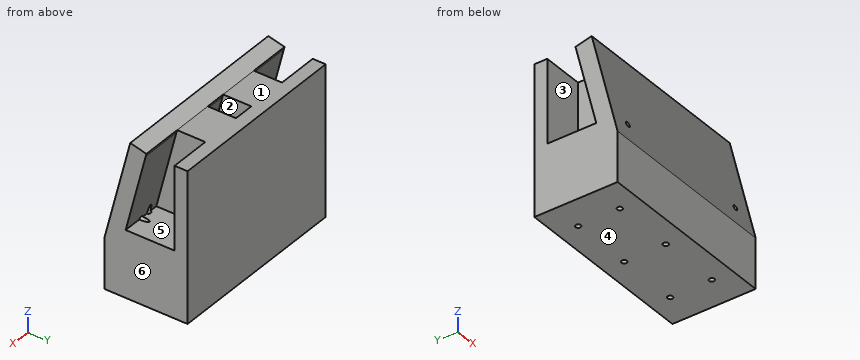
Autodesk Inventor part; units mm, degrees
ref_plane "作業平面1" through (45, 0, 0) normal (-1, 0, 0) x (0, 0, 1)
ref_plane "YZ Plane" through (0, 0, 0) normal (1, 0, 0) x (0, 1, 0)
ref_plane "XZ Plane" through (0, 0, 0) normal (0, 1, 0) x (-1, 0, 0)
sketch "スケッチ1" plane through (0, 0, 0) normal (1, 0, 0) x (0, 1, 0)
  line L0 (0, 0) -> (19.3538, 77.6237)
  line L1 (0, 0) -> (80, 0) construction
  line L2 (19.3538, 77.6237) -> (20.7024, 0.3614)
  line L3 (20.7024, 0.3614) -> (0, 0)
  line L4 (0, 0) -> (20.7024, 0.3614)
  line L5 (0, 0) -> (40, 0)
  line L6 (40, 0) -> (40, 77.6237)
  line L7 (40, 77.6237) -> (19.3538, 77.6237)
  dimension "d0" = 80
  dimension "d1" = 76
  dimension "d2" = 15
  dimension "d44" = 40
extrude "押し出し1" add sketch "スケッチ1" along normal blind 90
sketch "スケッチ2" plane through (0, 0, 0) normal (0, -0.9703, 0.2419) x (1, 0, 0)
  line L0 (0, 80) -> (10, 80)
  line L1 (10, 80) -> (10, 70)
  line L2 (10, 70) -> (0, 70)
  line L3 (0, 70) -> (0, 80)
  line L4 (90, 80) -> (80, 80)
  line L5 (80, 80) -> (80, 70)
  line L6 (80, 70) -> (90, 70)
  line L7 (90, 70) -> (90, 80)
  line L8 (90, 0) -> (80, 0)
  line L9 (80, 0) -> (80, 10)
  line L10 (80, 10) -> (90, 10)
  line L11 (90, 10) -> (90, 0)
  line L12 (0, 0) -> (10, 0)
  line L13 (10, 0) -> (10, 10)
  line L14 (10, 10) -> (0, 10)
  line L15 (0, 10) -> (0, 0)
  dimension "d5" = 10
  dimension "d6" = 10
  dimension "d7" = 10
  dimension "d8" = 10
  dimension "d9" = 10
  dimension "d10" = 10
  dimension "d11" = 10
  dimension "d12" = 10
hole "穴1" at (10, 16.9345, 67.9207) at (10, 2.4192, 9.703) at (80, 2.4192, 9.703) at (80, 16.9345, 67.9207) direction (0, 0.9703, -0.2419) diameter 2.5 depth 20 tip angle 118
sketch "スケッチ4" plane through (90, 0, 0) normal (1, 0, 0) x (0, 0, -1)
  line L0 (-77.6237, 19.3538) -> (0, 0)
  line L1 (0, 0) -> (0, 20.7055)
  line L2 (-8, 20.7055) -> (-8, 1.9946)
  line L3 (0, 12.7075) -> (-47.6322, 11.876)
  line L4 (-46.7187, 19.8932) -> (0, 8.2449)
  line L5 (-77.6237, 40) -> (-77.6237, 19.3538)
  line L6 (-46.7187, 19.8932) -> (-70.3029, 25.7734)
  line L7 (-70.3029, 25.7734) -> (-70.3029, 33.7734)
  line L8 (-70.3029, 33.7734) -> (-8, 33.7734)
  line L9 (-8, 33.7734) -> (-8, 20)
  point P0 (-16.7273, 12.4155)
  point P1 (-8, 12.5678)
  point P2 (-8, 10.2395)
  dimension "d34" = 8
  dimension "d36" = 8
  dimension "d45" = 8
ref_plane "作業平面1" through (45, 0, 0) normal (-1, 0, 0) x (0, 0, 1)
extrude "押し出し4" cut sketch "スケッチ4" against normal blind 45 contours L4 L6 L7 L8 L9 L2 L3 | L3 L2 L4
mirror "ミラー1" about plane through (45, 0, 0) normal (-1, 0, 0) of "押し出し4"
sketch "スケッチ6" plane through (0, 0, 0) normal (0, 0, -1) x (-1, 0, 0)
  line L0 (-90, 40) -> (-75, 40)
  line L1 (-75, 40) -> (-75, 30)
  line L2 (-75, 30) -> (-90, 30)
  line L3 (-90, 30) -> (-90, 40)
  line L4 (-90, 0) -> (-75, 0)
  line L5 (-75, 0) -> (-75, 10)
  line L6 (-75, 10) -> (-90, 10)
  line L7 (-90, 10) -> (-90, 0)
  line L8 (0, 40) -> (-15, 40)
  line L9 (-15, 40) -> (-15, 30)
  line L10 (-15, 30) -> (0, 30)
  line L11 (0, 30) -> (0, 40)
  line L12 (0, 0) -> (-15, 0)
  line L13 (-15, 0) -> (-15, 10)
  line L14 (-15, 10) -> (0, 10)
  line L15 (0, 10) -> (0, 0)
  point P0 (-45, 30)
  point P1 (-45, 10)
  dimension "d49" = 15
  dimension "d50" = 10
  dimension "d51" = 10
  dimension "d52" = 15
  dimension "d53" = 10
  dimension "d54" = 10
hole "穴3" at (45, 30, 0) at (45, 10, 0) at (15, 10, 0) at (15, 30, 0) at (75, 30, 0) at (75, 10, 0) direction (0, 0, 1) diameter 2.5 depth 8 tip angle 118
sketch "スケッチ7" plane through (90, 0, 0) normal (1, 0, 0) x (0, 0, -1)
  line L0 (-70.3029, 33.7734) -> (-8, 33.7734)
  line L1 (-8, 33.7734) -> (-8, 10.2395)
  line L2 (-8, 10.2395) -> (-70.3029, 25.7734)
  line L3 (-70.3029, 25.7734) -> (-70.3029, 33.7734)
  line L4 (0, 0) -> (0, 40)
  line L5 (0, 40) -> (-77.6237, 40)
  line L6 (-77.6237, 40) -> (-77.6237, 19.3538)
  line L7 (-77.6237, 19.3538) -> (0, 0)
ref_plane "作業平面2" through (70, 0, 0) normal (1, 0, 0) x (0, 0, -1)
sketch "スケッチ8" plane through (70, 0, 0) normal (1, 0, 0) x (0, 0, -1)
  line L0 (-5.9326, 37.4868) -> (-71.6084, 37.4868)
  line L1 (-71.6084, 37.4868) -> (-71.6084, 19.3326)
  line L2 (-28.0915, 7.5857) -> (-5.9326, 7.5857)
  line L3 (-5.9326, 7.5857) -> (-5.9326, 37.4868)
  line L4 (-28.0915, 7.5857) -> (-71.6084, 19.3326)
  point P0 (0, 0)
extrude "押し出し5" add sketch "スケッチ8" against normal blind 20
ref_plane "作業平面3" through (20, 0, 0) normal (-1, 0, 0) x (0, 0, 1)
sketch "スケッチ9" plane through (20, 0, 0) normal (-1, 0, 0) x (0, 0, 1)
  line L0 (5.473, 36.709) -> (72.4836, 36.709)
  line L1 (72.4836, 36.709) -> (72.4836, 22.6929)
  line L2 (20.9575, 8.6767) -> (5.473, 8.6767)
  line L3 (5.473, 8.6767) -> (5.473, 36.709)
  line L4 (20.9575, 8.6767) -> (72.4836, 22.6929)
  point P0 (0, 0)
extrude "押し出し6" add sketch "スケッチ9" against normal blind 20
sketch "スケッチ10" plane through (0, 0, 0) normal (-1, 0, 0) x (0, 0, 1)
  line L0 (77.6237, 40) -> (48.0044, 40)
  line L1 (50.463, 10.3528) -> (77.6237, 10.3528)
  line L2 (77.6237, 10.3528) -> (77.6237, 40)
  line L3 (70.3029, 25.7734) -> (8, 10.2395)
  line L4 (77.6237, 19.3538) -> (0, 0)
  line L5 (48.0044, 20.2137) -> (49.9397, 12.4514)
  line L6 (49.9397, 12.4514) -> (50.463, 10.3528)
  line L7 (48.0044, 40) -> (48.0044, 20.2137)
  line L8 (47.6237, 11.8739) -> (47.6237, 10.3528)
  dimension "d68" = 30
extrude "押し出し7" cut sketch "スケッチ10" against normal blind 100
sketch "スケッチ11" plane through (0, 0, 0) normal (0, 0, -1) x (-1, 0, 0)
  circle A0 centre (-75, 30) radius 1.25
  circle A1 centre (-15, 10) radius 1.25
  circle A2 centre (-45, 30) radius 1.25
  circle A3 centre (-45, 10) radius 1.25
  circle A4 centre (-15, 30) radius 1.25
  circle A5 centre (-75, 10) radius 1.25
  line L0 (0, 0) -> (0, 40)
  line L1 (0, 40) -> (-90, 40)
  line L2 (-90, 0) -> (-90, 40)
  line L3 (0, 0) -> (-90, 0)
extrude "押し出し8" add sketch "スケッチ11" along normal blind 24
sketch "スケッチ12" plane through (0, 0, -24) normal (0, 0, -1) x (-1, 0, 0)
  circle A0 centre (-75, 10) radius 1.25
  circle A1 centre (-45, 10) radius 1.25
  circle A2 centre (-15, 10) radius 1.25
extrude "押し出し9" cut sketch "スケッチ12" against normal blind 37
properties part number "知能ロボコン土台1.1"
Here's how the part is built. I have some questions about the finished solid (model axes, mm). Face numbers are marked on the shaded views. A direction names the side the tool comes from. Give positions to 0.01 mm unless a question says otherwise; leave off trailing zeros. Loops run counter-clockwise (first coordinate to the right, second up) from the corner with the lowest first, then second, coordinate; pieces in that order, holes last. Notation, with made-up numbers: M 84,-25 L 99,-25 A29 ccw 99,14 Z; hole C 38.5,36 d2. An arc over 180 degrees is marked long. Put each result on its own line as item: value. Start each with the question number.
(1) If we mould it in two halves opening along Z, with no side actions, what happens to the marked faces 4, 5 and 6? For each: +Z half, -Z half, draft (parallel to the pull), parting line (faces both ways), or undercut.
(2) Will these pins go through, and if not, where does the flat tip stop? pin 1 Ø2 at (x, y) = (75, 10) entering from -Z; pin 2 Ø10 at (x, y) = (47, 29) entering from +Z; pin 3 Ø7 at (y, z) = (24.5, 24) entering from -X; pin 4 Ø2 at (x, y) = (45, 30) entering from +Z.
(3) I need wall thicknesses on line 1 along Y through (x, z) = (15, -13.5); line 2 along X through (y, z) = (30, -7); line 3 along X through (y, z) = (25, 16.5). Which ranges of each line are inside material? Lowest first, please. Write a range as [from, to].
(4) I want a section at C-C on x = 53. Please give me the cut outline in (y, z).
(5) For the marked faces 1, 2 and 3, which set-ups out of +Z, -Z, +X, -X, +Y, -Y let a thin tool reach every point of the face, with its end or its side?
(6) I want a section at D-D on y = 17.5. State how many separate pieces and enclosed holes the cut face has, then the cut area to 3 significant figures.
(7) I want a section at B-B on z = 35.5. Please give me the cut outline in (x, y).
Answer block:
1. face 4: -Z half
1. face 5: undercut
1. face 6: draft
2. pin 1: z = 13
2. pin 2: z = 48
2. pin 3: x = 20
2. pin 4: through
3. line 1: [0, 8.75], [11.25, 28.75], [31.25, 40]
3. line 2: [0, 13.75], [16.25, 43.75], [46.25, 73.75], [76.25, 90]
3. line 3: [20, 40], [50, 70]
4. outline: M 0,-24 L 40,-24 L 40,48 L 20.21,48 L 12.45,49.94 L 0,0 Z
5. face 1: +Z, +X, -X, +Y
5. face 2: none
5. face 3: +Z, -X
6. separate pieces: 1
6. enclosed holes: 3
6. area: 5,080 mm^2
7. outline: M 0,8.85 L 90,8.85 L 90,17.1 L 70,17.1 L 70,33.77 L 90,33.77 L 90,40 L 0,40 L 0,33.77 L 20,33.77 L 20,17.1 L 0,17.1 Z; hole M 40,17.1 L 50,17.1 L 50,33.77 L 40,33.77 Z
